Part model, mm, in its own coordinate system. Coordinates: 2 decimals unless noted, no trailing zeros. Loops run counter-clockwise (first coordinate to the right, second up) from the corner with the lowest first, then second, coordinate; pieces in that order, holes last. Notation, with made-up numbers: M -18,13 L 26,13 A36 cw 26,49 Z; hole C 0,1 d9. An arc over 180 degrees is marked long. Answer as a JSON object with one key per item and string values. Group by question number.
1. Saw through at B-B on z = 4.75. Write the cut outline in (x, y), then the cut area to 3 significant figures.
2. Saw through at A-A on y = 0. Write the cut outline in (x, z).
3. Saw through at C-C on x = -20. Write the cut outline in (y, z).
4. Saw through at D-D on x = 0. Write the cut outline in (y, z), then the cut area to 3 significant figures.
5. Drill centre lines: L1, parallel to X at y = 0, z = 6; L2, parallel to Y at x = -20, z = 2.25; L3, parallel to Y at x = 0, z = 3.5. Where is each one in solid material? Low to high.
6. Mould opens along X. For faces 1 (the face through (-2.23, -2.43, 5.07)), 2 (the face through (-1, 3.4, 0)), 3 (the face through (-75, 0, 5)) say: released by +X, released by -X, zero draft, split by the parting line, or undercut.
Autodesk Inventor part; units mm, degrees
ref_plane "YZ Plane" through (0, 0, 0) normal (1, 0, 0) x (0, 1, 0)
ref_plane "XZ Plane" through (0, 0, 0) normal (0, 1, 0) x (-1, 0, 0)
ref_plane "XY Plane" through (0, 0, 0) normal (0, 0, 1) x (1, 0, 0)
sketch "Skizze1" plane through (0, 0, 0) normal (0, 0, 1) x (1, 0, 0)
  line L0 (75, 7.5) -> (-75, 7.5)
  line L1 (-75, 7.5) -> (-75, -7.5)
  line L2 (-75, -7.5) -> (75, -7.5)
  line L3 (75, -7.5) -> (75, 7.5)
  line L4 (75, 7.5) -> (-75, -7.5) construction
  line L5 (-75, 7.5) -> (75, -7.5) construction
  line L6 (-20, 0) -> (20, 0) construction
  point P0 (0, 0)
  point P1 (0, 0)
  point P2 (0, 0)
  dimension "d0" = 40
  dimension "d1" = 15
  dimension "d2" = 150
extrude "Extrusion1" add sketch "Skizze1" along normal blind 10
hole "Bohrung1" at (-20, 0, 0) at (20, 0, 0) direction (0, 0, 1) diameter 4.5 end through all
hole "Bohrung2" at (0, 0, 0) direction (0, 0, 1) diameter 6.6 end through all
properties part number "ParallelMecha_V2_BaseFormation_Proximal"
Outcome:
{
 "1": {"outline": "M -75,-7.5 L 75,-7.5 L 75,7.5 L -75,7.5 Z; hole C -20,0 d4.5; hole C 0,0 d6.6; hole C 20,0 d4.5", "area": "2,180 mm²"},
 "2": {"outline": "M -75,0 L -22.25,0 L -22.25,10 L -75,10 Z; M -17.75,0 L -3.3,0 L -3.3,10 L -17.75,10 Z; M 3.3,0 L 17.75,0 L 17.75,10 L 3.3,10 Z; M 22.25,0 L 75,0 L 75,10 L 22.25,10 Z"},
 "3": {"outline": "M -7.5,0 L -2.25,0 L -2.25,10 L -7.5,10 Z; M 2.25,0 L 7.5,0 L 7.5,10 L 2.25,10 Z"},
 "4": {"outline": "M -7.5,0 L -3.3,0 L -3.3,10 L -7.5,10 Z; M 3.3,0 L 7.5,0 L 7.5,10 L 3.3,10 Z", "area": "84.0 mm²"},
 "5": {"L1": "x = -75 to -22.25, -17.75 to -3.3, 3.3 to 17.75, 22.25 to 75", "L2": "y = -7.5 to -2.25, 2.25 to 7.5", "L3": "y = -7.5 to -3.3, 3.3 to 7.5"},
 "6": {"face 1": "undercut", "face 2": "zero draft", "face 3": "released by -X"}
}
